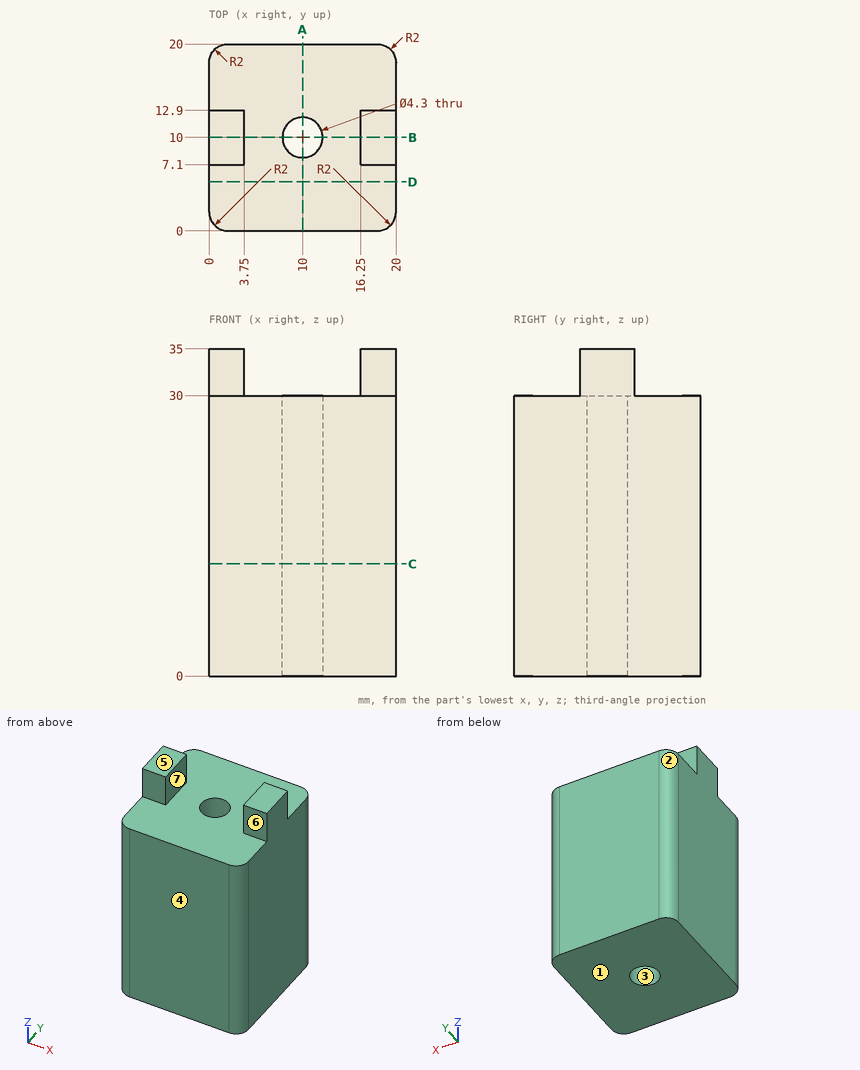
Could you check a few things on this drawing? It's one solid part, dimensions in mm from its lowest x, y, z. A direction names the side the tool comes from. Coordinates: 2 decimals unless noted, no trailing zeros. Loops run counter-clockwise (first coordinate to the right, second up) from the corner with the lowest first, then second, coordinate; pieces in that order, holes last.
1. For P1, Ø1, axis at x = 11.5, y = 13, coming from the +Z side; P2, Ø1.1, axis at x = 1.5, z = 32.5, coming from the +Y side; P3, Ø1.1, axis at x = 2.5, z = 32, coming from the -Y side, each with a flat end and sliding along its axis, tell me the tip position at first contact or that it passes through.
2. Imagine slicing it at D-D (y = 5.25). Please give me the cut outline in (x, z), and give its area (3 significant figures).
3. We'd pull the mould along Y, two halves only. Please class the marked faces 1, 2, 3 and 4: released by +Y, released by -Y, zero draft, split by the parting line, or undercut.
4. Imagine slicing it at A-A (x = 10). Please give me the cut outline in (y, z).
5. Imagine slicing it at C-C (z = 12). Please give me the cut outline in (x, y), and give its area (3 significant figures).
6. I need wall thicknesses on L1, parallel to Y at x = 10, z = 15.75; L2, parallel to Z at x = 4.25, y = 7.5; L3, parallel to X at y = 10.25, z = 7. Which ranges of each line are inside material? Lowest first, please.
7. Imagine slicing it at B-B (y = 10). Please give me the cut outline in (x, z).
8. For the marked faces 5, 6 and 7, which set-ups out of +Z, -Z, +X, -X, +Y, -Y let a thin tool reach every point of the face, with its end or its side?
Computed values:
1. P1: stops at z = 30
1. P2: stops at y = 12.9
1. P3: stops at y = 7.1
2. outline: (0, 0) - (20, 0) - (20, 30) - (0, 30) - close
2. area: 600 mm2
3. face 1: zero draft
3. face 2: released by +Y
3. face 3: undercut
3. face 4: released by -Y
4. outline: (0, 0) - (7.85, 0) - (7.85, 30) - (0, 30) - close; (12.15, 0) - (20, 0) - (20, 30) - (12.15, 30) - close
5. outline: (0, 2) arc R2 ccw to (2, 0) - (18, 0) arc R2 ccw to (20, 2) - (20, 18) arc R2 ccw to (18, 20) - (2, 20) arc R2 ccw to (0, 18) - close; hole circle Ø4.3 at (10, 10)
5. area: 382 mm2
6. L1: y = 0 to 7.85, 12.15 to 20
6. L2: z = 0 to 30
6. L3: x = 0 to 7.86, 12.14 to 20
7. outline: (0, 0) - (7.85, 0) - (7.85, 30) - (3.75, 30) - (3.75, 35) - (0, 35) - close; (12.15, 0) - (20, 0) - (20, 35) - (16.25, 35) - (16.25, 30) - (12.15, 30) - close
8. face 5: +Z, +X, -X, +Y, -Y
8. face 6: +Z, +X, -X, -Y
8. face 7: +Z, +Y, -Y
